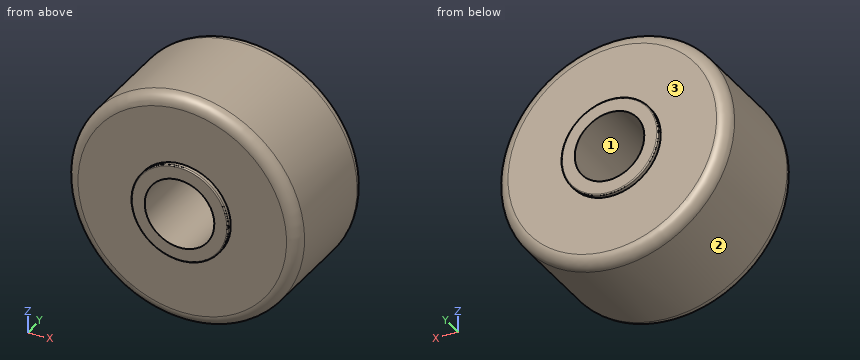
```python
from build123d import *

# Parameters (mm, degrees)
FILLET1_R = 5.08
FILLET2_R = 0.508


with BuildPart() as part:
    # Sketch1 → Revolve1 (revolve)
    with BuildSketch(Plane(origin=(0, 0, 0), x_dir=(0, 0, -1), z_dir=(1, 0, 0)), mode=Mode.PRIVATE) as revolve1_sk:
        Polygon((21.2725, -25.781), (21.2725, -27.94), (15.2527, -27.94), (15.2527, 27.94), (21.2725, 27.94), (21.2725, 25.781), (50.8, 25.781), (50.8, -25.781), align=None)
    revolve(revolve1_sk.sketch.rotate(Axis((0, 25.781, 0), (0, -1, 0)), 180), axis=Axis((0, 25.781, 0), (0, -1, 0)))

    # Fillet1
    fillet1_edges = [part.edges().sort_by_distance(p)[0] for p in [
        (0, -25.781, -50.8),
        (0, 25.781, -50.8),
    ]]
    fillet(fillet1_edges, radius=FILLET1_R)

    # Fillet2
    fillet2_edges = [part.edges().sort_by_distance(p)[0] for p in [
        (0, -27.94, -21.2725),
        (0, 27.94, -21.2725),
    ]]
    fillet(fillet2_edges, radius=FILLET2_R)


solid = part.part
```
Read the model definition and answer for the solid it produces. Units are mm, in the model's axes. Face numbers are marked on the shaded views. Coordinates: 2 decimals unless noted, no trailing zeros. Write each loop counter-clockwise with the first axis right and the second up, starting at its lowest first coordinate (ties: lowest second). Pieces come first, ordered by that corner, then holes. Notation, with made-up numbers: (48, -29) - (65, -29) arc R23 ccw to (65, -3) - close; hole circle Ø5 at (2, 24.25). An arc over 180 degrees is marked (long way). Answer as a JSON object with one key per item and string values. Group by question number.
1. Consider L1, parallel to X at y = 15.5, z = 0; L2, parallel to X at y = 8.5, z = 0.5; L3, parallel to Y at x = -29, z = -3.5. Determine where each line is inside the solid, lowest interval first. Write a range as [from, to].
2. Each of these flat-tipped pins is pushed along its axis until it touches: P1, Ø8, axis at x = 6, y = 8, coming from the +Z side; P2, Ø2, axis at x = -34, z = 25.5, coming from the +Y side; P3, Ø6, axis at y = -19.5, z = -21.5, coming from the +X side. Where does it stop, or does it pass through?
3. A cutting plane is placed at B-B (z = 0). Determine the outline of the cut face in (x, y).
4. A cutting plane is placed at C-C (y = -1). Determine the outline of the cut face in (x, z), plus the area to 3 significant figures.
5. The mould has two halves that part along Z. Classify the marked faces 1, 2 and 3: +Z half, -Z half, draft (parallel to the pull), parting line (faces both ways), or undercut.
6. A cutting plane is placed at A-A (x = 0). Determine the outline of the cut face in (y, z), plus the area to 3 significant figures.
Worked out:
{
 "1": {"L1": "x = [-50.8, -15.25], [15.25, 50.8]", "L2": "x = [-50.8, -15.24], [15.24, 50.8]", "L3": "y = [-25.78, 25.78]"},
 "2": {"P1": "stops at z = 50.76", "P2": "stops at y = 25.78", "P3": "stops at x = 47.31"},
 "3": {"outline": "(-50.8, -20.7) arc R5.08 ccw to (-45.72, -25.78) - (-21.27, -25.78) - (-21.27, -27.43) arc R0.51 ccw to (-20.76, -27.94) - (-15.25, -27.94) - (-15.25, 27.94) - (-20.76, 27.94) arc R0.51 ccw to (-21.27, 27.43) - (-21.27, 25.78) - (-45.72, 25.78) arc R5.08 ccw to (-50.8, 20.7) - close; (15.25, -27.94) - (20.76, -27.94) arc R0.51 ccw to (21.27, -27.43) - (21.27, -25.78) - (45.72, -25.78) arc R5.08 ccw to (50.8, -20.7) - (50.8, 20.7) arc R5.08 ccw to (45.72, 25.78) - (21.27, 25.78) - (21.27, 27.43) arc R0.51 ccw to (20.76, 27.94) - (15.25, 27.94) - close"},
 "4": {"outline": "circle Ø101.6 at (0, 0); hole circle Ø30.51 at (0, 0)", "area": "7,380 mm²"},
 "5": {"face 1": "undercut", "face 2": "parting line", "face 3": "draft"},
 "6": {"outline": "(-27.94, -20.76) arc R0.51 ccw to (-27.43, -21.27) - (-25.78, -21.27) - (-25.78, -45.72) arc R5.08 ccw to (-20.7, -50.8) - (20.7, -50.8) arc R5.08 ccw to (25.78, -45.72) - (25.78, -21.27) - (27.43, -21.27) arc R0.51 ccw to (27.94, -20.76) - (27.94, -15.25) - (-27.94, -15.25) - close; (-27.94, 15.25) - (27.94, 15.25) - (27.94, 20.76) arc R0.51 ccw to (27.43, 21.27) - (25.78, 21.27) - (25.78, 45.72) arc R5.08 ccw to (20.7, 50.8) - (-20.7, 50.8) arc R5.08 ccw to (-25.78, 45.72) - (-25.78, 21.27) - (-27.43, 21.27) arc R0.51 ccw to (-27.94, 20.76) - close", "area": "3,700 mm²"}
}
